CAD build for the part. Positions are in the model's coordinates, mm. A direction names the side the tool comes from. Give positions to 0.01 mm unless a question says otherwise; leave off trailing zeros. Order: outer loops, then holes, each group sorted by start corner. A loop starts at its lowest first (then second) coordinate and runs counter-clockwise, first axis right, second up. Notation, with made-up numbers: M 37.25,39 L 55.25,39 A8 ccw 55.25,48 Z; hole C 34,85.5 d10. An arc over 180 degrees is marked long. Put each result on its own line as item: value. Start each with the question number.
1) Drill centre lines: line 1 (Y direction, x = -15, z = 1.7); line 2 (X direction, y = 0.5, z = 10.25); line 3 (Y direction, x = 14.5, z = 2.5). Where is each one in solid material? Low to high. Write a range as [from, to].
2) Pin check, flat tips, straight feed: pin 1 (0.8 mm diameter, centred on x = -12.5, y = 6.5, fed in from +Z); pin 2 (5 mm diameter, centred on y = -0.5, z = 9, fed in from -X); pin 3 (1.5 mm diameter, centred on x = 12, y = 0, fed in from +Z). Stop position of each tip, or through.
3) Two-plate mould, pull along X, no slides. Class faces 1 (the face through (-12, 4, 8)), 2 (the face through (-17, 2, 2)), 3 (the face through (-12.5, -4.5, 4.2)): released by +X, released by -X, zero draft, split by the parting line, or undercut.
4) Cut at C-C (x = 15). Write the cut outline in (y, z), and give its area (3 significant figures).
5) Tool access for faces 4 (the face through (12.5, -4.5, 4.2)), 5 (the face through (13, 3, 7)), 6 (the face through (14, 9, 15)): list every direction of +Z, -Z, +X, -X, +Y, -Y with a clear straight run to the whole face (end or side of a thin tool).
6) Cut at D-D (z = 9). Write the cut outline in (x, y).
7) Cut at B-B (y = -6). Write the cut outline in (x, z), and give its area (3 significant figures).
8) Cut at A-A (z = 7). Write the cut outline in (x, y).
```python
from build123d import *

# Parameters (mm, degrees)
F0_W     = 34
F0_H     = 20
F0_R     = 1.25
F1_DEPTH = 3
F2_W     = 5
F2_H     = 1.5
F3_DEPTH = 12
F4_W     = 1
F4_H     = 13
F5_DEPTH = 10
F6_SIZE  = 7.5
F8_D     = 1


# Not quite as in the source:
# - a feature names something its author has since deleted; it is built from what else it names


with BuildPart() as f1:
    # F0 (on Top) → F1 (new body)
    with BuildSketch(Plane.XY):
        Rectangle(F0_W, F0_H)
        with Locations((-15, -6)):
            Circle(F0_R, mode=Mode.SUBTRACT)
        with Locations((15, -6)):
            Circle(F0_R, mode=Mode.SUBTRACT)
        with Locations((-15, 6)):
            Circle(F0_R, mode=Mode.SUBTRACT)
        with Locations((15, 6)):
            Circle(F0_R, mode=Mode.SUBTRACT)
    extrude(amount=F1_DEPTH)

    # F2 (on face) → F3 (join)
    with BuildSketch(Plane.XY.offset(3)):
        with Locations((-14.5, 9.25)):
            Rectangle(F2_W, F2_H)
        with Locations((14.5, 9.25)):
            Rectangle(F2_W, F2_H)
    extrude(amount=F3_DEPTH)

    # F4 (on face) → F5 (join)
    with BuildSketch(Plane.XY.offset(3)):
        with Locations((-12.5, 2)):
            Rectangle(F4_W, F4_H)
        with Locations((12.5, 2)):
            Rectangle(F4_W, F4_H)
    extrude(amount=F5_DEPTH)

    # F6
    f6_edges = [f1.edges().sort_by_distance(p)[0] for p in [
        (-12.5, -4.5, 13),
        (12.5, -4.5, 13),
    ]]
    chamfer(f6_edges, length=F6_SIZE)

    # F8 (through all)
    with Locations(Plane(origin=(0, 10, 0), x_dir=(-1, 0, 0), z_dir=(0, 1, 0))):
        with Locations((13.75, 9), (-13.75, 9)):
            Hole(F8_D / 2)


solid = f1.part
```
Solution:
1. line 1: [-10, -7.25], [-4.75, 4.75], [7.25, 10]
1. line 2: [-13, -12], [12, 13]
1. line 3: [-10, -7.15], [-4.85, 4.85], [7.15, 10]
2. pin 1: z = 13
2. pin 2: x = -13
2. pin 3: z = 10.75
3. face 1: undercut
3. face 2: released by -X
3. face 3: zero draft
4. outline: M -10,0 L -7.25,0 L -7.25,3 L -10,3 Z; M -4.75,0 L 4.75,0 L 4.75,3 L -4.75,3 Z; M 7.25,0 L 10,0 L 10,15 L 8.5,15 L 8.5,3 L 7.25,3 Z
4. area: 63.0 mm²
5. face 4: +Z, +X, -X, -Y
5. face 5: +Z, +X, -Y
5. face 6: +Z, +X, -X, +Y, -Y
6. outline: M -17,8.5 L -14.25,8.5 L -14.25,10 L -17,10 Z; M -13.25,8.5 L -13,8.5 L -13,-1 L -12,-1 L -12,10 L -13.25,10 Z; M 12,-1 L 13,-1 L 13,8.5 L 13.25,8.5 L 13.25,10 L 12,10 Z; M 14.25,8.5 L 17,8.5 L 17,10 L 14.25,10 Z
7. outline: M -17,0 L -16.25,0 L -16.25,3 L -17,3 Z; M -13.75,0 L 13.75,0 L 13.75,3 L -13.75,3 Z; M 16.25,0 L 17,0 L 17,3 L 16.25,3 Z
7. area: 87.0 mm²
8. outline: M -17,8.5 L -13,8.5 L -13,-3 L -12,-3 L -12,10 L -17,10 Z; M 12,-3 L 13,-3 L 13,8.5 L 17,8.5 L 17,10 L 12,10 Z
